The model under review builds one solid part; all positions refer to its coordinate system, in mm. Face numbers are marked on the shaded views. A direction names the side the tool comes from. Coordinates: 2 decimals unless noted, no trailing zeros. Use one line per item in the form item = value.
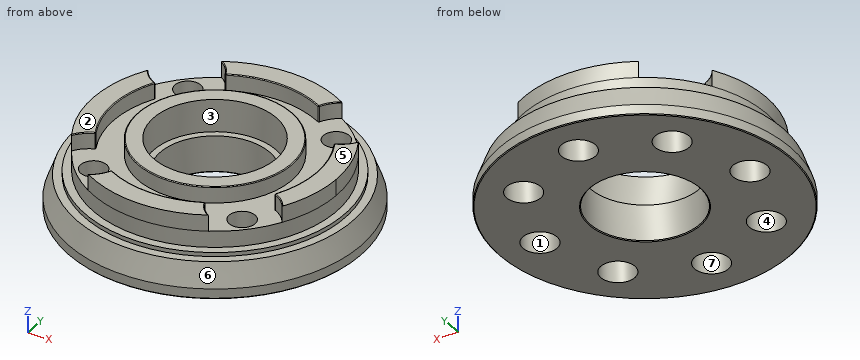
from build123d import *

# Parameters (mm, degrees)
BOSS_EXTRUDE1_DEPTH     = 2
BOSS_EXTRUDE1_2_DEPTH   = 2
BOSS_EXTRUDE1_3_DEPTH   = 2
BOSS_EXTRUDE1_4_DEPTH   = 2
SKETCH1_R               = 9.5
SKETCH1_R_2             = 7.5625
BOSS_EXTRUDE1_5_DEPTH   = 2
BOSS_EXTRUDE2_START     = -2
SKETCH2_R               = 15
BOSS_EXTRUDE2_DEPTH     = 2
FILLET1_R               = 0.1
FILLET2_R               = 0.1
SKETCH4_R               = 16
BOSS_EXTRUDE3_DEPTH     = 0.5
SKETCH5_R               = 18
BOSS_EXTRUDE4_DEPTH     = 4
CUT_EXTRUDE2_DEPTH      = 26.850531909
CUT_EXTRUDE2_DEPTH_BACK = 26.850531909
SKETCH3_R               = 1.6
SKETCH6_R               = 2.1
CUT_EXTRUDE3_DEPTH      = 4
SKETCH7_R               = 2.1
CUT_EXTRUDE4_DEPTH      = 4
SKETCH8_R               = 6.75
MIDDLE_CUTOUT_DEPTH     = 7
CHAMFER1_SIZE           = 0.1
CUT_EXTRUDE6_START      = -2
SKETCH9_R               = 7.5625
CUT_EXTRUDE6_DEPTH      = 2
CHAMFER2_SIZE           = 1
CHAMFER2_SIZE2          = 2.747477419


with BuildPart() as part:
    # Sketch1 → Boss-Extrude1 (new body)
    with BuildSketch(Plane.XY):
        with BuildLine():
            ThreePointArc((5.795745748, 11.075167323), (6.469207051, 12.179609111), (7.456549067, 13.01537076))
            ThreePointArc((7.456549067, 13.01537076), (0, 15), (-7.456549067, 13.01537076))
            ThreePointArc((-7.456549067, 13.01537076), (-6.469207051, 12.179609111), (-5.795745748, 11.075167323))
            ThreePointArc((-5.795745748, 11.075167323), (0, 12.5), (5.795745748, 11.075167323))
        make_face()
    extrude(amount=BOSS_EXTRUDE1_DEPTH)



with BuildPart() as body_2:
    # Sketch1 → Boss-Extrude1 2 (new body)
    with BuildSketch(Plane.XY):
        with BuildLine():
            ThreePointArc((13.01537076, -7.456549067), (14.495353762, -3.858071967), (15, 0))
            ThreePointArc((15, 0), (14.495353762, 3.858071967), (13.01537076, 7.456549067))
            ThreePointArc((13.01537076, 7.456549067), (12.179609111, 6.469207051), (11.075167323, 5.795745748))
            ThreePointArc((11.075167323, 5.795745748), (12.5, 0), (11.075167323, -5.795745748))
            ThreePointArc((11.075167323, -5.795745748), (12.179609111, -6.469207051), (13.01537076, -7.456549067))
        make_face()
    extrude(amount=BOSS_EXTRUDE1_2_DEPTH)


with BuildPart() as body_3:
    # Sketch1 → Boss-Extrude1 3 (new body)
    with BuildSketch(Plane.XY):
        with BuildLine():
            ThreePointArc((-7.456549067, -13.01537076), (0, -15), (7.456549067, -13.01537076))
            ThreePointArc((7.456549067, -13.01537076), (6.469207051, -12.179609111), (5.795745748, -11.075167323))
            ThreePointArc((5.795745748, -11.075167323), (0, -12.5), (-5.795745748, -11.075167323))
            ThreePointArc((-5.795745748, -11.075167323), (-6.469207051, -12.179609111), (-7.456549067, -13.01537076))
        make_face()
    extrude(amount=BOSS_EXTRUDE1_3_DEPTH)


with BuildPart() as body_4:
    # Sketch1 → Boss-Extrude1 4 (new body)
    with BuildSketch(Plane.XY):
        with BuildLine():
            ThreePointArc((-11.075167323, 5.795745748), (-12.179609111, 6.469207051), (-13.01537076, 7.456549067))
            ThreePointArc((-13.01537076, 7.456549067), (-15, 0), (-13.01537076, -7.456549067))
            ThreePointArc((-13.01537076, -7.456549067), (-12.179609111, -6.469207051), (-11.075167323, -5.795745748))
            ThreePointArc((-11.075167323, -5.795745748), (-12.5, 0), (-11.075167323, 5.795745748))
        make_face()
    extrude(amount=BOSS_EXTRUDE1_4_DEPTH)


with BuildPart() as body_5:
    # Sketch1 → Boss-Extrude1 5 (new body)
    with BuildSketch(Plane.XY):
        Circle(SKETCH1_R)
        Circle(SKETCH1_R_2, mode=Mode.SUBTRACT)
    extrude(amount=BOSS_EXTRUDE1_5_DEPTH)


with BuildPart() as part_1:
    add(part.part)

    add(body_2.part)  # Boss-Extrude2 merges body 2

    add(body_3.part)  # Boss-Extrude2 merges body 3

    add(body_4.part)  # Boss-Extrude2 merges body 4

    add(body_5.part)  # Boss-Extrude2 merges body 5
    # Sketch2 → Boss-Extrude2 (add)
    with BuildSketch(Plane.XY.offset(BOSS_EXTRUDE2_START)):
        with Locations(Location((0, 0, 0), (0, 0, 150.191461703))):
            Circle(SKETCH2_R)
    extrude(amount=BOSS_EXTRUDE2_DEPTH)

    # Fillet1
    fillet1_edges = [part_1.edges().sort_by_distance(p)[0] for p in [
        (11.075167323, 5.795745748, 1),
        (11.075167323, -5.795745748, 1),
        (5.795745748, -11.075167323, 1),
        (-5.795745748, -11.075167323, 1),
        (-11.075167323, -5.795745748, 1),
        (-11.075167323, 5.795745748, 1),
        (5.795745748, 11.075167323, 1),
        (-5.795745748, 11.075167323, 1),
    ]]
    fillet(fillet1_edges, radius=FILLET1_R)

    # Fillet2
    fillet2_edges = [part_1.edges().sort_by_distance(p)[0] for p in [
        (6.504180663, 12.219925602, 2),
        (12.219925602, -6.504180663, 2),
        (-6.504180663, -12.219925602, 2),
        (-12.219925602, 6.504180663, 2),
        (-9.5, 0, 2),
        (0, -12.5, 2),
        (6.504180663, -12.219925602, 2),
        (5.779303749, -11.119440592, 2),
        (-5.779303749, -11.119440592, 2),
        (12.5, 0, 2),
        (12.219925602, 6.504180663, 2),
        (11.119440592, 5.779303749, 2),
        (11.119440592, -5.779303749, 2),
        (0, 12.5, 2),
        (-6.504180663, 12.219925602, 2),
        (-5.779303749, 11.119440592, 2),
        (5.779303749, 11.119440592, 2),
        (-12.5, 0, 2),
        (-12.219925602, -6.504180663, 2),
        (-11.119440592, -5.779303749, 2),
        (-11.119440592, 5.779303749, 2),
    ]]
    fillet(fillet2_edges, radius=FILLET2_R - 0.0001)  # a hair under: the kernel refuses the full size

    # Sketch4 → Boss-Extrude3 (add)
    with BuildSketch(Plane(origin=(0, 0, -2), x_dir=(-1, 0, 0), z_dir=(0, 0, -1))):
        Circle(SKETCH4_R)
    extrude(amount=BOSS_EXTRUDE3_DEPTH)

    # Sketch5 → Boss-Extrude4 (add)
    with BuildSketch(Plane(origin=(0, 0, -2.5), x_dir=(-1, 0, 0), z_dir=(0, 0, -1))):
        Circle(SKETCH5_R)
    extrude(amount=BOSS_EXTRUDE4_DEPTH)

    # Sketch3 → Cut-Extrude2 (cut, two sides: drawn at the far end of the back side and taken through both)
    with BuildSketch(Plane(origin=(0, 0, -2), x_dir=(-1, 0, 0), z_dir=(0, 0, -1)).offset(-CUT_EXTRUDE2_DEPTH_BACK)):
        with Locations((-9.192388155, 9.192388155)):
            Circle(SKETCH3_R)
        with Locations((9.192388155, 9.192388155)):
            Circle(SKETCH3_R)
        with Locations((9.192388155, -9.192388155)):
            Circle(SKETCH3_R)
        with Locations((-9.192388155, -9.192388155)):
            Circle(SKETCH3_R)
    extrude(amount=CUT_EXTRUDE2_DEPTH + CUT_EXTRUDE2_DEPTH_BACK, mode=Mode.SUBTRACT)

    # Sketch6 → Cut-Extrude3 (cut)
    with BuildSketch(Plane(origin=(0, 0, -6.5), x_dir=(-1, 0, 0), z_dir=(0, 0, -1))):
        with Locations((-9.192388155, 9.192388155)):
            Circle(SKETCH6_R)
        with Locations((9.192388155, 9.192388155)):
            Circle(SKETCH6_R)
        with Locations((9.192388155, -9.192388155)):
            Circle(SKETCH6_R)
        with Locations((-9.192388155, -9.192388155)):
            Circle(SKETCH6_R)
    extrude(amount=-CUT_EXTRUDE3_DEPTH, mode=Mode.SUBTRACT)

    # Sketch7 → Cut-Extrude4 (cut)
    with BuildSketch(Plane(origin=(0, 0, -6.5), x_dir=(-1, 0, 0), z_dir=(0, 0, -1))):
        with Locations((0, 13)):
            Circle(SKETCH7_R)
        with Locations((13, 0)):
            Circle(SKETCH7_R)
        with Locations((0, -13)):
            Circle(SKETCH7_R)
        with Locations((-13, 0)):
            Circle(SKETCH7_R)
    extrude(amount=-CUT_EXTRUDE4_DEPTH, mode=Mode.SUBTRACT)

    # Sketch8 → Middle Cutout (cut)
    with BuildSketch(Plane.XY):
        Circle(SKETCH8_R)
    extrude(amount=-MIDDLE_CUTOUT_DEPTH, mode=Mode.SUBTRACT)

    # Chamfer1
    chamfer1_edges = [part_1.edges().sort_by_distance(p)[0] for p in [
        (18, 0, -6.5),
        (-6.75, 0, -6.5),
    ]]
    chamfer(chamfer1_edges, length=CHAMFER1_SIZE)

    # Sketch9 → Cut-Extrude6 (cut)
    with BuildSketch(Plane.XY.offset(CUT_EXTRUDE6_START)):
        Circle(SKETCH9_R)
    extrude(amount=CUT_EXTRUDE6_DEPTH, mode=Mode.SUBTRACT)

    # Chamfer2
    chamfer2_edges = [part_1.edges().sort_by_distance(p)[0] for p in [
        (18, 0, -2.5),
    ]]
    chamfer2_side = [part_1.faces().sort_by_distance(p)[0] for p in [
        (17.490883118, 0, -2.5),
    ]]
    chamfer(chamfer2_edges, length=CHAMFER2_SIZE, length2=CHAMFER2_SIZE2, reference=chamfer2_side[0])


solid = part_1.part
Item 1: Tool access review of the marked faces 1, 2 and 3: name each direction out of +Z, -Z, +X, -X, +Y, -Y from which nothing blocks a thin tool from reaching the whole face with its end or side.
Results found:
face_1 = -Z
face_2 = +Z, +X, -X, +Y, -Y
face_3 = +Z
Item 2: Clearance check with flat-ended pins moving along their axes: pin 1 (6.5 mm diameter, centred on x = -9.19, y = -9.19, fed in from -Z); pin 2 (2 mm diameter, centred on x = -8.5, y = 9, fed in from -Z); pin 3 (4 mm diameter, centred on y = 9, z = 0.5, fed in from +X). State where each tip first meets the part, or that it passes through.
Results found:
pin_1 = -6.5
pin_2 = -2.5
pin_3 = 13.27
Item 3: To check wall thickness, follow L1, parallel to Y at x = 7.5, z = -4.25; L2, parallel to Z at x = -12, y = -10; L3, parallel to Z at x = -10.5, y = 4. State the ranges of each line that lie inside material, in increasing order. Write a range as from..to.
Results found:
L1 = -15.96..-10.44, -7.95..7.95, 10.44..15.96
L2 = -6.5..-2
L3 = -6.5..0
Item 4: Draft analysis for pull direction X (two halves, no side actions). For the marked faces 4, 5, 6 and 7, state which applies: released by +X, released by -X, zero draft, split by the parting line, or undercut.
Results found:
face_4 = undercut
face_5 = zero draft
face_6 = split by the parting line
face_7 = undercut
